```python
from build123d import *

# Parameters (mm, degrees)
RECPAT_COUNT = 2
RECPAT_ANGLE = 90


with BuildPart() as part:
    # Fillet1: read off the stored shape, not the designer's step
    # Fillet1 outline → Fillet1 (revolve)
    with BuildSketch(Plane.YX):
        with BuildLine():
            Line((2, 3.3), (2, 8.1))
            Line((2, 8.1), (0, 8.1))
            Line((0, 8.1), (0, 0))
            ThreePointArc((0, 0), (2.027933458, 0.324444488), (3.853420198, 1.265388956))
            ThreePointArc((3.853420198, 1.265388956), (3.961271902, 1.392873227), (4, 1.555305874))
            Line((4, 1.555305874), (4, 3.1))
            Line((4, 3.1), (2.2, 3.1))
            ThreePointArc((2.2, 3.1), (2.058578644, 3.158578644), (2, 3.3))
        make_face()
    revolve(axis=Axis((0, 0, 0), (1, 0, 0)))

    # Sketch3 → Recess section 0
    with BuildSketch(Plane(origin=(0, 0, 0), x_dir=(0, 0, -1), z_dir=(1, 0, 0))):
        with BuildLine():
            Line((0.515, -2.15), (-0.515, -2.15))
            Line((-0.515, -2.15), (-0.515, 2.15))
            Line((-0.515, 2.15), (0.515, 2.15))
            Line((0.515, 2.15), (0.515, -2.15))
        make_face()
    # Sketch4 → Recess section 1
    with BuildSketch(Plane(origin=(2.34, 0, 0), x_dir=(0, 0, -1), z_dir=(1, 0, 0))):
        with BuildLine():
            Line((0.515, -0.983319232), (-0.515, -0.983319232))
            Line((-0.515, -0.983319232), (-0.515, 0.983319232))
            Line((-0.515, 0.983319232), (0.515, 0.983319232))
            Line((0.515, 0.983319232), (0.515, -0.983319232))
        make_face()
    recess = loft(mode=Mode.SUBTRACT)

    # RecPat: Recess ×2 about axis
    recpat_axis = Axis((0, 0, 0), (1, 0, 0))
    for i in range(1, RECPAT_COUNT):
        add(recess.rotate(recpat_axis, i * RECPAT_ANGLE / (RECPAT_COUNT - 1)), mode=Mode.SUBTRACT)

    # RecCorSke → RecessCore (revolve, cut)
    with BuildSketch(Plane.XY, mode=Mode.PRIVATE) as recesscore_sk:
        Polygon((0, 0), (0, 1.01462874), (2.34, 0.851), (2.616506661, 0), align=None)
    revolve(recesscore_sk.sketch.rotate(Axis((-3.175, 0, 0), (1, 0, 0)), 90), axis=Axis((-3.175, 0, 0), (1, 0, 0)), mode=Mode.SUBTRACT)


solid = part.part
```
Here's how the part is built. I have some questions about the finished solid (model axes, mm). A direction names the side the tool comes from. Give positions to 0.01 mm unless a question says otherwise; leave off trailing zeros. Order: outer loops, then holes, each group sorted by start corner. A loop starts at its lowest first (then second) coordinate and runs counter-clockwise, first axis right, second up. Notation, with made-up numbers: M 50.25,70.5 L 72.25,70.5 A26 cw 72.25,102.5 Z; hole C 0,-9 d3. An arc over 180 degrees is marked long. Use a Markdown table: item, result. Add a question column.
1. If we mould it in two halves opening along Z, with no side actions, what happens to faces 1 (the cylindrical face through (2.338, -0.867, -3.905)), 2 (the flat face through (8.1, 0, 0)), 3 (the flat face through (1.3, -1.5, 0))? For each: +Z half, -Z half, draft (parallel to the pull), parting line (faces both ways), or undercut.
2. For pin 1 Ø1 at (x, y) = (6, 1.5) entering from +Z; pin 2 Ø1 at (x, z) = (6, 2) entering from -Y; pin 3 Ø2 at (y, z) = (-2.5, 0.5) entering from -X, each with a flat end and sliding along its axis, tell me the tip position at first contact or that it passes through.
3. On a 3-axis mill with a long thin cutter (end or side, diameter ignored), from which of +Z, -Z, +X, -X, +Y, -Y can I reach the whole of each face in a straight line? I mean faces 4 (the flat face through (1.3, 0, -1.5)), 5 (the flat face through (3.1, 2, -2)). Say none if no direction works.
4. Suppose I cut it at A-A (x = 4.5). List the corners of the cut face in (y, z) for me.
5. Suppose I cut it at B-B (x = 2.75). List the corners of the cut face in (y, z) for me, and give its area (3 significant figures).
6. I need wall thicknesses on probe 1 along Y at (x, z) = (7.25, -0.25); probe 2 along Z at (x, y) = (7, 0); probe 3 along Y at (x, z) = (2, -0.75) (3 decimals). Which ranges of each line are inside material? Lowest first, please. Write a range as from..to.
Results list:
| question | item | result |
|---|---|---|
| 1 | face 1 | parting line |
| 1 | face 2 | draft |
| 1 | face 3 | undercut |
| 2 | pin 1 | stops at z = 1.73 |
| 2 | pin 2 | stops at y = -1.32 |
| 2 | pin 3 | stops at x = 0.2 |
| 3 | face 4 | -X |
| 3 | face 5 | +X |
| 4 | outline | C 0,0 d4 |
| 5 | outline | C 0,0 d8 |
| 5 | area | 50.3 mm² |
| 6 | probe 1 | y = -1.98..1.98 |
| 6 | probe 2 | z = -2..2 |
| 6 | probe 3 | y = -3.929..-0.515, 0.515..3.929 |
